Autodesk Inventor part; units mm, degrees
ref_plane "YZ Plane" through (0, 0, 0) normal (1, 0, 0) x (0, 1, 0)
ref_plane "XZ Plane" through (0, 0, 0) normal (0, 1, 0) x (-1, 0, 0)
ref_plane "XY Plane" through (0, 0, 0) normal (0, 0, 1) x (1, 0, 0)
sketch "Sketch1" plane through (0, 0, 0) normal (0, 0, 1) x (1, 0, 0)
  line L0 (-6, 4) -> (6, 4)
  line L1 (6, 4) -> (6, -4)
  line L2 (6, -4) -> (-6, -4)
  line L3 (-6, -4) -> (-6, 4)
  line L4 (-6, 4) -> (6, -4) construction
  line L5 (6, 4) -> (-6, -4) construction
  line L6 (-6, 2.0607) -> (-4.9393, 1)
  line L7 (-6, 2.0607) -> (-4.5, 2.0607) construction
  line L8 (-4.9393, 1) -> (-6, -0.0607)
  line L9 (0, 4) -> (0, -4) construction
  line L10 (6, 2.0607) -> (4.9393, 1)
  line L11 (4.9393, 1) -> (6, -0.0607)
  point P0 (0, 0)
  point P1 (6, -0.0607)
  point P2 (6, 2.0607)
  dimension "d0" = 12
  dimension "d1" = 8
  dimension "d2" = 45
  dimension "d3" = 3
  dimension "d4" = 1.5
extrude "Extrusion1" add sketch "Sketch1" along normal mid plane 300 contours L0 L1 L10 L11 L2 L3 L8 L6
sketch "Sketch2" plane through (-6, 4, 150) normal (0, 1, 0) x (1, 0, 0)
  point P0 (6, 150)
  point P1 (6, 150)
  point P2 (6, 162.5)
  dimension "d17" = 12.5
hole "Hole1" at (0, 4, -12.5) direction (0, -1, 0) diameter 3.5 end through all counterbore diameter 6 counterbore depth 4.5
pattern_linear "Rectangular Pattern1" count 12 spacing 25 along (0, 0, 1) of "Hole1" first direction both ways yes
sketch "Sketch3" plane through (-6, 4, 150) normal (0, 1, 0) x (1, 0, 0)
  circle A0 centre (6, 12.5) radius 3
  circle A1 centre (6, 287.5) radius 3
  point P0 (6, 150)
hole "Hole2" at (0, 4, 137.5) at (0, 4, -137.5) direction (0, -1, 0) diameter 6 end through all
properties part number "MGN15 Rail" material "Stainless Steel, 440C"
Design review of the part built by this model. Coordinates are the model's own, in mm. A direction names the side the tool comes from. Give positions to 0.01 mm unless a question says otherwise; leave off trailing zeros. Order: outer loops, then holes, each group sorted by start corner. A loop starts at its lowest first (then second) coordinate and runs counter-clockwise, first axis right, second up. Notation, with made-up numbers: (26, -14) - (55, -14) arc R15 cw to (55, 1) - close; hole circle Ø7 at (66, 88.25). An arc over 180 degrees is marked (long way). Use a Markdown table: item, result. Add a question column.
(1) Wall thickness on probe 1 along Z at (x, y) = (-2.25, -1); probe 2 along Z at (x, y) = (-2, -0.75); probe 3 along X at (y, z) = (0.45, 87.5): over which ranges is each line inside the solid? List them lowest first. Write a range as [from, to].
(2) Add section C-C on z = 80. Give the boundary of the cut face in (x, y).
(3) Add section B-B on z = 137.5. Give the boundary of the cut face in (x, y).
(4) Clearance check with flat-ended pins moving along their axes: P1, Ø1.8, axis at x = 0, z = 38.5, coming from the +Y side; P2, Ø3, axis at x = 0, z = -37.5, coming from the -Y side. State where each tip first meets the part, or that it passes through.
(5) Mouldability with a two-part tool opening along X and no side actions: class faces 3 (the face through (-0.1, 1.7, 34.5)), 4 (the face through (0, 0, 150)) as +X half, -X half, draft (parallel to the pull), parting line (faces both ways), or undercut.
(6) Add section A-A on y = -1.75. Give the number of separate pieces and of enclosed holes in the cut face, then the cut area to 3 significant figures.
(7) Machinability: for faces 1 (the face through (2, -0.5, -88)), 2 (the face through (-0.9, -0.06, -134.64)), which of the approach directions +Z, -Z, +X, -X, +Y, -Y give a long, thin tool a straight path to every point of the face, cutting with its end or side? Answer none if there is none.
Report:
| question | item | result |
|---|---|---|
| 1 | probe 1 | z = [-150, -139.48], [-135.52, 135.52], [139.48, 150] |
| 1 | probe 2 | z = [-150, -139.74], [-135.26, 135.26], [139.74, 150] |
| 1 | probe 3 | x = [-5.49, -3], [3, 5.49] |
| 2 | outline | (-6, -4) - (6, -4) - (6, -0.06) - (4.94, 1) - (6, 2.06) - (6, 4) - (-6, 4) - (-6, 2.06) - (-4.94, 1) - (-6, -0.06) - close |
| 3 | outline | (-6, -4) - (-3, -4) - (-3, 4) - (-6, 4) - (-6, 2.06) - (-4.94, 1) - (-6, -0.06) - close; (3, -4) - (6, -4) - (6, -0.06) - (4.94, 1) - (6, 2.06) - (6, 4) - (3, 4) - close |
| 4 | P1 | stops at y = -0.5 |
| 4 | P2 | passes through |
| 5 | face 3 | undercut |
| 5 | face 4 | draft |
| 6 | separate pieces | 1 |
| 6 | enclosed holes | 12 |
| 6 | area | 3,450 mm² |
| 7 | face 1 | +Y |
| 7 | face 2 | +Y, -Y |
